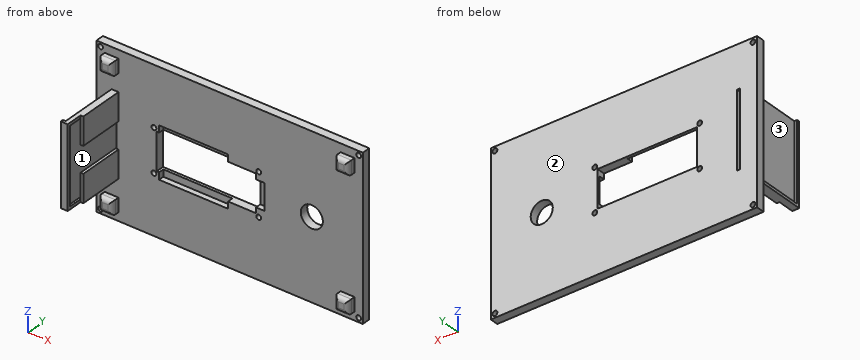
from build123d import *

# Parameters (mm, degrees)
SKETCH1_W            = 193
SKETCH1_H            = 116.5
SKETCH1_R            = 1.75
SKETCH1_R_2          = 8
SKETCH1_W_2          = 72
SKETCH1_H_2          = 27
SKETCH1_W_3          = 2
SKETCH1_H_3          = 55
BOSS_EXTRUDE1_DEPTH  = 6
SKETCH3_W            = 10
SKETCH3_H            = 10
BOSS_EXTRUDE3_DEPTH  = 10
SKETCH5_W            = 2
SKETCH5_H            = 55
BOSS_EXTRUDE4_DEPTH  = 6
SKETCH6_W            = 181
SKETCH6_H            = 104.5
CUT_EXTRUDE1_DEPTH   = 4
SKETCH7_W            = 1.5
SKETCH7_H            = 55
BOSS_EXTRUDE5_DEPTH  = 44.75
SKETCH8_W            = 2
SKETCH8_H            = 55
CUT_EXTRUDE2_DEPTH   = 42.25
SKETCH10_W           = 6
SKETCH10_H           = 19
CUT_EXTRUDE3_DEPTH   = 4
FILLET3_R            = 3
SKETCH12_W           = 55
SKETCH12_H           = 2
BOSS_EXTRUDE6_DEPTH  = 1.5
SKETCH14_W           = 3
SKETCH14_H           = 44.75
BOSS_EXTRUDE7_DEPTH  = 2
SKETCH15_W           = 3
SKETCH15_H           = 44.75
BOSS_EXTRUDE8_DEPTH  = 2
BOSS_EXTRUDE9_DEPTH  = 2
SKETCH18_W           = 20
SKETCH18_H           = 32.75
BOSS_EXTRUDE10_DEPTH = 2
SKETCH19_W           = 50
SKETCH19_H           = 37
CUT_EXTRUDE7_DEPTH   = 4


with BuildPart() as part:
    # Sketch1 → Boss-Extrude1 (new body)
    with BuildSketch(Plane(origin=(0, 0, 0), x_dir=(1, 0, 0), z_dir=(0, 1, 0))):
        with Locations((22.87983871, -17.078434096)):
            Rectangle(SKETCH1_W, SKETCH1_H)
        with Locations(Location((-31.988235573, -1.578434096, 0), (0, 0, 270))):
            Circle(SKETCH1_R, mode=Mode.SUBTRACT)
        with Locations(Location((-31.988235573, -32.578434096, 0), (0, 0, 270))):
            Circle(SKETCH1_R, mode=Mode.SUBTRACT)
        with Locations(Location((44.011764427, -1.578434096, 0), (0, 0, 270))):
            Circle(SKETCH1_R, mode=Mode.SUBTRACT)
        with Locations(Location((44.011764427, -32.578434096, 0), (0, 0, 270))):
            Circle(SKETCH1_R, mode=Mode.SUBTRACT)
        with Locations(Location((-70.62016129, -72.328434096, 0), (0, 0, 270))):
            Circle(SKETCH1_R, mode=Mode.SUBTRACT)
        with Locations(Location((-70.62016129, 38.171565904, 0), (0, 0, 270))):
            Circle(SKETCH1_R, mode=Mode.SUBTRACT)
        with Locations(Location((116.37983871, -72.328434096, 0), (0, 0, 270))):
            Circle(SKETCH1_R, mode=Mode.SUBTRACT)
        with Locations(Location((116.37983871, 38.171565904, 0), (0, 0, 270))):
            Circle(SKETCH1_R, mode=Mode.SUBTRACT)
        with Locations(Location((82.450678359, -17.078434096, 0), (0, 0, 270))):
            Circle(SKETCH1_R_2, mode=Mode.SUBTRACT)
        with Locations((6.011764427, -17.078434096)):
            Rectangle(SKETCH1_W_2, SKETCH1_H_2, mode=Mode.SUBTRACT)
        with Locations((-47.331266899, -17.078434096)):
            Rectangle(SKETCH1_W_3, SKETCH1_H_3, mode=Mode.SUBTRACT)
    extrude(amount=BOSS_EXTRUDE1_DEPTH)

    # Sketch3 → Boss-Extrude3 (add)
    with BuildSketch(Plane.XZ):
        with Locations((-62.62016129, 64.328434096)):
            Rectangle(SKETCH3_W, SKETCH3_H)
        with Locations((-62.62016129, -30.171565904)):
            Rectangle(SKETCH3_W, SKETCH3_H)
        with Locations((108.37983871, -30.171565904)):
            Rectangle(SKETCH3_W, SKETCH3_H)
        with Locations((108.37983871, 64.328434096)):
            Rectangle(SKETCH3_W, SKETCH3_H)
    extrude(amount=BOSS_EXTRUDE3_DEPTH)

    # Sketch5 → Boss-Extrude4 (add)
    with BuildSketch(Plane.XZ):
        with Locations((-47.331266899, 17.078434096)):
            Rectangle(SKETCH5_W, SKETCH5_H)
    extrude(amount=-BOSS_EXTRUDE4_DEPTH)

    # Sketch6 → Cut-Extrude1 (cut)
    with BuildSketch(Plane.XZ.offset(10)):
        with Locations((22.87983871, 17.078434096)):
            Rectangle(SKETCH6_W, SKETCH6_H)
    extrude(amount=-CUT_EXTRUDE1_DEPTH, mode=Mode.SUBTRACT)

    # Sketch7 → Boss-Extrude5 (add)
    with BuildSketch(Plane.XZ):
        with Locations((-61.87016129, 17.078434096)):
            Rectangle(SKETCH7_W, SKETCH7_H)
    extrude(amount=BOSS_EXTRUDE5_DEPTH)

    # Sketch8 → Cut-Extrude2 (cut)
    with BuildSketch(Plane.XZ):
        with Locations((-60.12016129, 17.078434096)):
            Rectangle(SKETCH8_W, SKETCH8_H)
    extrude(amount=-CUT_EXTRUDE2_DEPTH, mode=Mode.SUBTRACT)

    # Sketch10 → Cut-Extrude3 (cut)
    with BuildSketch(Plane.XZ):
        with Locations((45.011764427, 17.078434096)):
            Rectangle(SKETCH10_W, SKETCH10_H)
    extrude(amount=-CUT_EXTRUDE3_DEPTH, mode=Mode.SUBTRACT)

    # Fillet3
    fillet3_edges = [part.edges().sort_by_distance(p)[0] for p in [
        (-67.62016129, -6, 64.328434096),
        (-67.62016129, -6, -30.171565904),
        (-62.62016129, -6, -35.171565904),
        (108.37983871, -6, -35.171565904),
        (-62.62016129, -6, 69.328434096),
        (108.37983871, -6, 69.328434096),
        (113.37983871, -6, -30.171565904),
        (113.37983871, -6, 64.328434096),
        (-62.62016129, -6, 59.328434096),
        (-57.62016129, -6, 64.328434096),
        (103.37983871, -6, 64.328434096),
        (108.37983871, -6, 59.328434096),
        (108.37983871, -6, -25.171565904),
        (103.37983871, -6, -30.171565904),
        (-57.62016129, -6, -30.171565904),
        (-62.62016129, -6, -25.171565904),
    ]]
    fillet(fillet3_edges, radius=FILLET3_R)

    # Sketch12 → Boss-Extrude6 (add)
    with BuildSketch(Plane(origin=(-61.12016129, 0, 0), x_dir=(0, 0, -1), z_dir=(1, 0, 0))):
        with Locations((-17.078434096, -43.75)):
            Rectangle(SKETCH12_W, SKETCH12_H)
    extrude(amount=BOSS_EXTRUDE6_DEPTH)

    # Sketch14 → Boss-Extrude7 (add)
    with BuildSketch(Plane(origin=(0, 0, -10.421565904), x_dir=(-1, 0, 0), z_dir=(0, 0, -1))):
        with Locations((61.12016129, -22.375)):
            Rectangle(SKETCH14_W, SKETCH14_H)
    extrude(amount=BOSS_EXTRUDE7_DEPTH)

    # Sketch15 → Boss-Extrude8 (add)
    with BuildSketch(Plane.XY.offset(44.578434096)):
        with Locations((-61.12016129, -22.375)):
            Rectangle(SKETCH15_W, SKETCH15_H)
    extrude(amount=BOSS_EXTRUDE8_DEPTH)

    # Sketch16 → Boss-Extrude9 (add)
    with BuildSketch(Plane.ZY.offset(62.62016129)):
        Polygon((-10.421565904, 0), (-10.421565904, -42.75), (46.578434096, -42.75), (46.578434096, -44.75), (-12.421565904, -44.75), (-12.421565904, 0), align=None)
    extrude(amount=BOSS_EXTRUDE9_DEPTH)

    # Sketch18 → Boss-Extrude10 (add)
    with BuildSketch(Plane(origin=(-59.62016129, 0, 0), x_dir=(0, 0, -1), z_dir=(1, 0, 0))):
        with Locations((-36.578434096, -16.375)):
            Rectangle(SKETCH18_W, SKETCH18_H)
        with Locations((2.421565904, -16.375)):
            Rectangle(SKETCH18_W, SKETCH18_H)
    extrude(amount=BOSS_EXTRUDE10_DEPTH)

    # Sketch19 → Cut-Extrude7 (cut)
    with BuildSketch(Plane.XZ):
        with Locations((-3.238235573, 17.078434096)):
            Rectangle(SKETCH19_W, SKETCH19_H)
    extrude(amount=-CUT_EXTRUDE7_DEPTH, mode=Mode.SUBTRACT)


solid = part.part
For this review, take the finished solid that the model builds, in its own axes (mm). Face numbers are marked on the shaded views. Round coordinates to 2 decimals unless told otherwise and drop trailing zeros. Write each loop counter-clockwise with the first axis right and the second up, starting at its lowest first coordinate (ties: lowest second). Pieces come first, ordered by that corner, then holes. Notation, with made-up numbers: (31.25, -16.75) -> (73.25, -16.75) arc R17 cw to (73.25, 2.25) -> close; hole circle Ø1 at (-31.5, 86.25). An arc over 180 degrees is marked (long way). Use CSV: the item, a comma, the result in double quotes.
(1) Clearance check with flat-ended pins moving along their axes: P1, Ø2.5, axis at x = -60.5, y = -1, coming from the -Z side; P2, Ø16, axis at y = -16.5, z = 34, coming from the +X side; P3, Ø1, axis at x = -59, z = 38.5, coming from the -Y side; P4, Ø0.9, axis at x = 107, y = -1, coming from the -Z side. State where each tip first meets the part, or that it passes through.
Computed values:
P1,"z = -41.17"
P2,"x = -57.62"
P3,"y = -32.75"
P4,"z = -35.17"
(2) Consider section B-B, the plane x = 33. Give the boundary of the cut face in (y, z).
Computed values:
outline,"(0, -41.17) -> (6, -41.17) -> (6, 3.58) -> (0, 3.58) -> close; (0, 30.58) -> (6, 30.58) -> (6, 75.33) -> (0, 75.33) -> close"
(3) Consider section C-C, the plane z = 13.5. Give the boundary of the cut face in (x, y), plus the area to 3 significant figures.
Computed values:
outline,"(-73.62, 0) -> (-62.62, 0) -> (-62.62, -42.75) -> (-64.62, -42.75) -> (-64.62, -44.75) -> (-59.62, -44.75) -> (-59.62, -42.75) -> (-61.12, -42.75) -> (-61.12, 6) -> (-73.62, 6) -> close; (-59.12, 0) -> (-29.99, 0) -> (-29.99, 6) -> (-59.12, 6) -> close; (42.01, 4) -> (48.01, 4) -> (48.01, 0) -> (75.3, 0) -> (75.3, 6) -> (42.01, 6) -> close; (89.61, 0) -> (119.38, 0) -> (119.38, 6) -> (89.61, 6) -> close"
area,"678 mm²"
(4) To check wall thickness, follow L1, parallel to X at y = -17.5, z = -3; L2, parallel to Z at x = 39, y = 2.5; L3, parallel to Y at x = 75, z = 50.5. State the ranges of each line that lie inside material, in increasing order. Write a range as [from, to].
Computed values:
L1,"[-62.62, -61.12], [-59.62, -57.62]"
L2,"[-41.17, 3.58], [30.58, 75.33]"
L3,"[0, 6]"
(5) Consider section A-A, the plane z = 39.5. Give the boundary of the cut face in (x, y), plus the area to 3 significant figures.
Computed values:
outline,"(-73.62, 0) -> (-62.62, 0) -> (-62.62, -42.75) -> (-64.62, -42.75) -> (-64.62, -44.75) -> (-59.62, -44.75) -> (-59.62, -42.75) -> (-61.12, -42.75) -> (-61.12, 6) -> (-73.62, 6) -> close; (-59.62, -32.75) -> (-57.62, -32.75) -> (-57.62, 0) -> (119.38, 0) -> (119.38, 6) -> (-59.12, 6) -> (-59.12, 0) -> (-59.62, 0) -> close"
area,"1,290 mm²"
(6) Draft analysis for pull direction X (two halves, no side actions). For the marked faces 1, 2 and 3, state which applies: +X half, -X half, draft (parallel to the pull), parting line (faces both ways), or undercut.
Computed values:
face 1,"undercut"
face 2,"draft"
face 3,"-X half"
(7) Consider section D-D, the plane y = -25. Give the boundary of the cut face in (x, z).
Computed values:
outline,"(-64.62, -12.42) -> (-57.62, -12.42) -> (-57.62, 7.58) -> (-59.62, 7.58) -> (-59.62, -10.42) -> (-61.12, -10.42) -> (-61.12, 44.58) -> (-59.62, 44.58) -> (-59.62, 26.58) -> (-57.62, 26.58) -> (-57.62, 46.58) -> (-62.62, 46.58) -> (-62.62, -10.42) -> (-64.62, -10.42) -> close"
